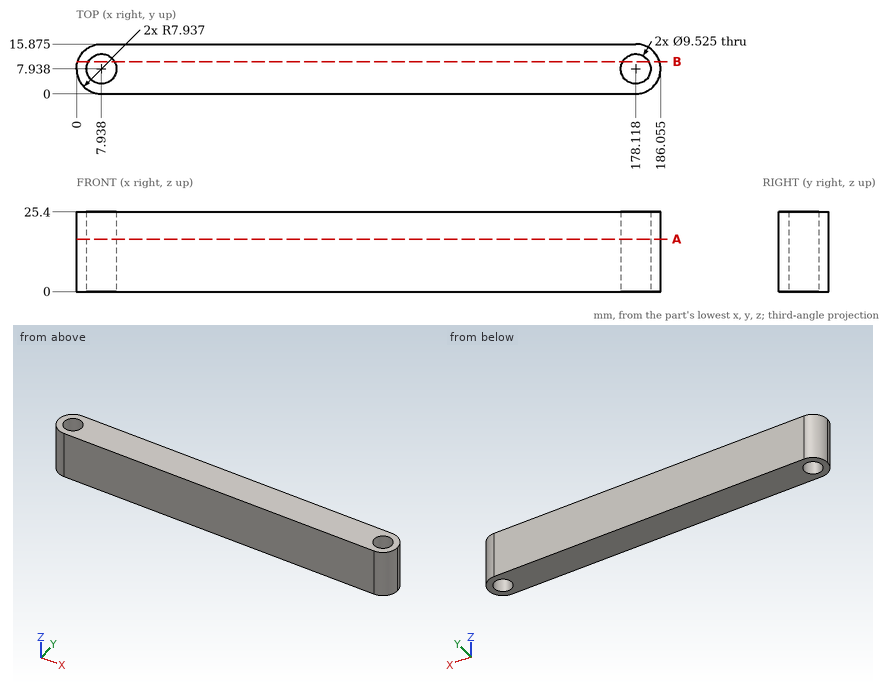
For this review, use the dimensioned drawing (mm, ordinates from the lowest corner) and the shaded views. Round coordinates to 2 decimals unless told otherwise and drop trailing zeros. Loops run counter-clockwise (first coordinate to the right, second up) from the corner with the lowest first, then second, coordinate; pieces in that order, holes last. Notation, with made-up numbers: M 23.25,-33 L 32.25,-33 A22 ccw 32.25,-9 Z; hole C 53.5,79.5 d1. An arc over 180 degrees is marked long. Answer as a JSON object with one key per item and string values.
(1) Take a section at B-B on y = 10.25. Give the boundary of the cut face in (x, z) (1 decimal).
Resolved:
{"outline": "M 0.3,0 L 3.8,0 L 3.8,25.4 L 0.3,25.4 Z; M 12.1,0 L 174,0 L 174,25.4 L 12.1,25.4 Z; M 182.3,0 L 185.7,0 L 185.7,25.4 L 182.3,25.4 Z"}
(2) Take a section at A-A on z = 16.75. Count the separate pieces of the cut face and the enclosed holes in it, and give its area (3 significant figures).
Resolved:
{"separate pieces": "1", "enclosed holes": "2", "area": "2,760 mm²"}
(3) To check wall thickness, follow line 1 along X through (y, z) = (8.5, 17.5) (1 decimal); line 2 along X through (y, z) = (7.5, 2.75) (1 decimal); line 3 along Y through (x, z) = (178, 21.75) (1 decimal). State the ranges of each line that lie inside material, in increasing order.
Resolved:
{"line 1": "0 to 3.2, 12.7 to 173.4, 182.8 to 186", "line 2": "0 to 3.2, 12.7 to 173.4, 182.9 to 186", "line 3": "0 to 3.2, 12.7 to 15.9"}
